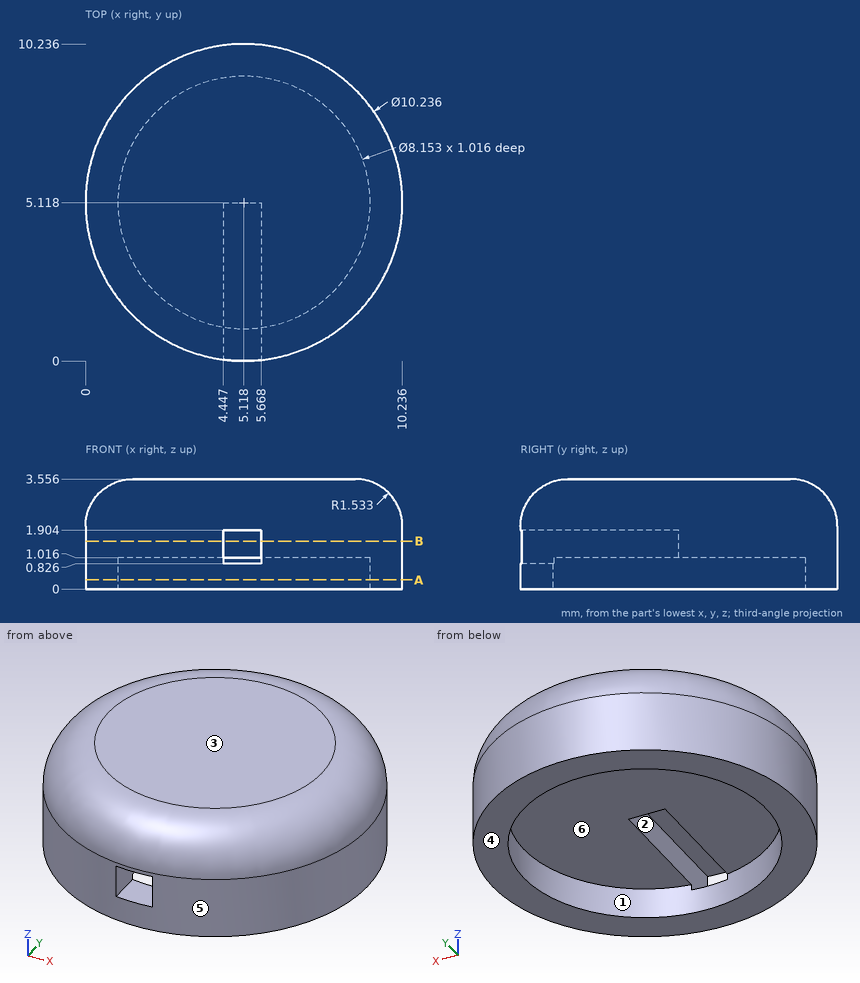
Input: dimensioned drawing with shaded views. Units: mm. Origin: part minimum x, y, z. A direction names the side the tool comes from. Give positions to 0.01 mm unless a question says otherwise; leave off trailing zeros. Order: outer loops, then holes, each group sorted by start corner. A loop starts at its lowest first (then second) coordinate and runs counter-clockwise, first axis right, second up. Notation, with made-up numbers: (11.25, 36) -> (55.25, 36) arc R33 ccw to (55.25, 72) -> close; hole circle Ø10 at (15, 46.25). An arc over 180 degrees is marked (long way). Answer as a JSON object with one key per item and string values.
Q1. Section B-B (z = 1.55). Output: boundary loops of the cut face in (x, y) (1 decimal).
Entries:
{"outline": "(4.4, 0) -> (4.4, 5.1) -> (5.7, 5.1) -> (5.7, 0) arc R5.1 ccw (long way) to start"}
Q2. Access query for the marked faces 1, 2 and 3. Directions: +Z, -Z, +X, -X, +Y, -Y. A direction counts if a zero-diameter tool reaches every point of the face in a straight line with its end or side. Return the directions, or none.
Entries:
{"face 1": "-Z", "face 2": "-Y", "face 3": "+Z, +X, -X, +Y, -Y"}
Q3. Draft query along Y for the marked faces 4, 5 and 6. Return one class per face: released by +Y, released by -Y, zero draft, split by the parting line, or undercut.
Entries:
{"face 4": "zero draft", "face 5": "split by the parting line", "face 6": "undercut"}
Q4. First-contact query: pin 1 (0.9 mm diameter, centred on x = 5, y = 0.5, fed in from +Z); pin 2 (2 mm diameter, centred on x = 2.5, z = 1, fed in from -Y); pin 3 (0.5 mm diameter, centred on y = 3.5, z = 1, fed in from +X). Flat tips, straight axial feed; report the tip coordinate or a pass-through.
Entries:
{"pin 1": "stops at z = 3.44", "pin 2": "stops at y = 0.26", "pin 3": "stops at x = 10.05"}
Q5. Section A-A (z = 0.3). Output: boundary loops of the cut face in (x, y) (1 decimal).
Entries:
{"outline": "circle Ø10.2 at (5.1, 5.1); hole circle Ø8.2 at (5.1, 5.1)"}
Q6. Material intervals for probe 1 along Z at (x, y) = (8, 3); probe 2 along X at (y, z) = (4.5, 0.9); probe 3 along X at (y, z) = (6, 0.7), sorted ascending.
Entries:
{"probe 1": "z = 1.02 to 3.56", "probe 2": "x = 0.04 to 1.09, 9.15 to 10.2", "probe 3": "x = 0.08 to 1.14, 9.1 to 10.16"}
